The model under review builds one solid part; all positions refer to its coordinate system, in mm. A direction names the side the tool comes from. Round coordinates to 2 decimals unless told otherwise and drop trailing zeros. Order: outer loops, then holes, each group sorted by start corner. A loop starts at its lowest first (then second) coordinate and runs counter-clockwise, first axis right, second up. Notation, with made-up numbers: (17.5, 50) -> (31.5, 50) arc R33 ccw to (31.5, 88) -> close; hole circle Ø4 at (53.5, 39). An arc over 180 degrees is marked (long way). Return JSON: item names as keys, results as strings. Group by question number.
Autodesk Inventor part; units mm, degrees
ref_plane "Work Plane1" through (1.525, 0, 0) normal (0, 0, 1) x (1, 0, 0)
ref_plane "YZ Plane" through (0, 0, 0) normal (1, 0, 0) x (0, 1, 0)
ref_plane "XZ Plane" through (0, 0, 0) normal (0, 1, 0) x (-1, 0, 0)
sketch "Sketch1" plane through (0, 0, 0) normal (0, 0, 1) x (1, 0, 0)
  line L0 (0, 5.0006) -> (0, 3.175)
  line L1 (50.8, 3.175) -> (69.85, 3.175)
  line L2 (69.85, 3.175) -> (69.85, 0)
  line L3 (69.85, 0) -> (-0.6351, 0)
  line L4 (-14.7321, 0) -> (83.947, 0)
  line L5 (-0.6351, 0) -> (-0.6351, 5.0006)
  line L6 (-0.6351, 5.0006) -> (0, 5.0006)
  line L7 (50.8, 3.175) -> (49.5299, 3.175)
  line L8 (49.5299, 3.175) -> (0, 3.175)
  line L9 (0, -1.0001) -> (0, 6.0007)
  dimension "d0" = 69.85
  dimension "d1" = 19.05
  dimension "d2" = 6.35
  dimension "d9" = 0.6351
  dimension "d10" = 10.0013
  dimension "d13" = 1.2701
  dimension "d14" = 6.35
revolve "Body" add sketch "Sketch1" angle 360 about axis through (69.85, 0, 0) along (-1, 0, 0)
sketch "Sketch2" plane through (-0.6351, 0, 0) normal (-1, 0, 0) x (0, 0, 1)
  line L0 (0, 6.4158) -> (5.5562, 3.2079)
  line L1 (5.5562, 3.2079) -> (5.5562, -3.2079)
  line L2 (5.5562, -3.2079) -> (0, -6.4158)
  line L3 (0, -6.4158) -> (-5.5562, -3.2079)
  line L4 (-5.5562, -3.2079) -> (-5.5562, 3.2079)
  line L5 (-5.5562, 3.2079) -> (0, 6.4158)
  point P0 (0, 0)
  point P1 (0, 0)
  dimension "d11" = 11.1125
extrude "Head" add sketch "Sketch2" along normal blind 3.3337
sketch "Sketch4" plane through (0, 0, 0) normal (0, 0, 1) x (1, 0, 0)
  line L0 (-3.9689, 5.5563) -> (-3.9689, 6.4158)
  line L1 (-3.9689, 6.4158) -> (-3.4726, 6.4158)
  line L2 (-3.4726, 6.4158) -> (-3.9689, 5.5563)
  line L3 (-4.6356, 0) -> (0.0317, 0)
  line L4 (-0.6351, 6.4158) -> (-3.9688, 6.4158)
  line L5 (-3.9688, 3.2079) -> (-3.9688, 6.4158)
  dimension "d5" = 30
  dimension "d19" = 11.1125
revolve "Chamfer1" cut sketch "Sketch4" angle 360 about axis through (-10, 0, 0) along (1, 0, 0)
thread "Thread"
chamfer "Chamfer2" distance 0.6875 distance2 1.2701 1 edges at (69.85, -3.175, 0) measured on face at (69.85, -0.7922, -0.7018)
ref_plane "Work Plane1" through (1.525, 0, 0) normal (0, 0, 1) x (1, 0, 0)
fillet "Fillet2" radius 0.635 1 edges at (0, -3.175, 0)
equation "\"d0\" = NLG"
equation "\"d1\" = GEL"
equation "\"d2\" = GD"
equation "\"d10\" = SD2"
equation "\"d14\" = BDM"
equation "\"d11\" = SW"
equation "\"d3\" = KOH - SD"
equation "\"d5\" = ANG1"
equation "\"d19\" = SW0"
equation "\"d63\" = R"
equation "\"d15\" = GEL"
equation "\"d6\" = -0.5 * SPD + 0.5 * GD"
equation "\"NLG\" = 69.85"
equation "\"GD\" = NND"
equation "\"BDM\" = 6.35"
equation "\"KOH\" = 3.96875"
equation "\"GEL\" = 19.05"
equation "\"SW\" = 11.1125"
equation "\"SW0\" = SW"
equation "\"SPD\" = 4.9751"
equation "\"SD2\" = 10.00125"
equation "\"SD\" = 0.635"
equation "\"ANG1\" = 30deg"
equation "\"GAL\" = 1.27"
equation "\"GUL\" = 1.27"
equation "\"R\" = 0.635"
equation "\"d62\" = -NLG - SD + GUL"
equation "\"THREADDIA\" = 6.35"
equation "\"TOA\" = 30deg"
equation "\"RR\" = 0.254"
equation "\"NND\" = 6.35"
equation "\"E0\" = 1.155 * SW"
equation "\"SLG\" = 0"
equation "\"GD1\" = 4.9751"
properties part number "ANSI B18.2.1 - 1/4-20 UNC - 2.75" material "Steel, Mild"
Item 1: Wall thickness on line 1 along X through (y, z) = (-2, -4); line 2 along X through (y, z) = (-2.75, -4.25); line 3 along Y through (x, z) = (65.5, -0.25): over which ranges is each line inside the solid? List them lowest first.
Item 2: Consider section A-A on x = 63.5. State the section outline as (y, z) points (3 decimals).
Item 3: For faces 1 (the face through (-3.85, 2.87, -5)), 2 (the face through (-0.3, -4, -3)), list the 3-axis set-ups (+Z, -Z, +X, -X, +Y, -Y) from which the entire face can be reached by the end or side of a thin tool; tool diameter is ignored.
Item 4: Insertion check: pin 1 Ø5 at (x, y) = (30, 0) entering from +Z (3 decimals); pin 2 Ø5 at (x, z) = (7.5, -3.5) entering from +Y; pin 3 Ø1.5 at (x, y) = (20, 5) entering from +Z; pin 4 Ø6 at (x, z) = (44, 0) entering from -Y (3 decimals). Each pin has a flat end and moves straight along its axis. Give the tip position at first contact, or say it passes through.
Values:
{
 "1": {"line 1": "-3.97 to 0", "line 2": "-3.97 to -0.64", "line 3": "-3.17 to 3.17"},
 "2": {"outline": "circle Ø6.35 at (0, 0)"},
 "3": {"face 1": "-Z, -X, +Y", "face 2": "+X"},
 "4": {"pin 1": "z = 3.175", "pin 2": "y = 3.01", "pin 3": "through", "pin 4": "y = -3.175"}
}
